```python
from build123d import *

# Parameters (mm, degrees)
SKETCH1_R           = 250
SKETCH1_R_2         = 20
BOSS_EXTRUDE1_DEPTH = 60


with BuildPart() as part:
    # Sketch1 → Boss-Extrude1 (new body)
    with BuildSketch(Plane(origin=(0, 0, 0), x_dir=(0, 0, -1), z_dir=(1, 0, 0))):
        Circle(SKETCH1_R)
        Circle(SKETCH1_R_2, mode=Mode.SUBTRACT)
        with BuildLine():
            Line((177.360116559, 68.142417438), (43.501893686, 24.649244324))
            ThreePointArc((43.501893686, 24.649244324), (29.389262615, 40.450849719), (10, 48.989794856))
            Line((10, 48.989794856), (10, 189.73665961))
            ThreePointArc((10, 189.73665961), (111.679197936, 153.713228931), (177.360116559, 68.142417438))
        make_face(mode=Mode.SUBTRACT)
        with BuildLine():
            Line((-10, 189.73665961), (-10, 48.989794856))
            ThreePointArc((-10, 48.989794856), (-29.389262615, 40.450849719), (-43.501893686, 24.649244324))
            Line((-43.501893686, 24.649244324), (-177.360116559, 68.142417438))
            ThreePointArc((-177.360116559, 68.142417438), (-111.679197936, 153.713228931), (-10, 189.73665961))
        make_face(mode=Mode.SUBTRACT)
        with BuildLine():
            Line((183.540456446, 49.121287113), (49.682233573, 5.628113998))
            ThreePointArc((49.682233573, 5.628113998), (47.552825815, -15.450849719), (36.885648873, -33.755724066))
            Line((36.885648873, -33.755724066), (119.614580282, -147.622329558))
            ThreePointArc((119.614580282, -147.622329558), (180.700738096, -58.713228931), (183.540456446, 49.121287113))
        make_face(mode=Mode.SUBTRACT)
        with BuildLine():
            Line((103.434240394, -159.378034603), (20.705308985, -45.511429112))
            ThreePointArc((20.705308985, -45.511429112), (0, -50), (-20.705308985, -45.511429112))
            Line((-20.705308985, -45.511429112), (-103.434240394, -159.378034603))
            ThreePointArc((-103.434240394, -159.378034603), (0, -190), (103.434240394, -159.378034603))
        make_face(mode=Mode.SUBTRACT)
        with BuildLine():
            Line((-119.614580282, -147.622329558), (-36.885648873, -33.755724066))
            ThreePointArc((-36.885648873, -33.755724066), (-47.552825815, -15.450849719), (-49.682233573, 5.628113998))
            Line((-49.682233573, 5.628113998), (-183.540456446, 49.121287113))
            ThreePointArc((-183.540456446, 49.121287113), (-180.700738096, -58.713228931), (-119.614580282, -147.622329558))
        make_face(mode=Mode.SUBTRACT)
    extrude(amount=BOSS_EXTRUDE1_DEPTH)


solid = part.part
```
Could you check a few things on this model? Use its own coordinates, in mm. A direction names the side the tool comes from. Coordinates: 2 decimals unless noted, no trailing zeros. Order: outer loops, then holes, each group sorted by start corner. A loop starts at its lowest first (then second) coordinate and runs counter-clockwise, first axis right, second up. Notation, with made-up numbers: M -1,-8.75 L 31,-8.75 A14 ccw 31,17.25 Z; hole C 41,14.5 d11. An arc over 180 degrees is marked long. Use one line per item in the form item = value. Start each with the question number.
1. We'd pull the mould along Y, two halves only. Please class faces 3 (the flat face through (0, 59, 3)), 4 (the flat face through (30, 118, -10)): +Y half, -Y half, draft (parallel to the pull), parting line (faces both ways), or undercut.
2. Suppose I cut it at B-B on x = 31.5. Write out the boundary of the cut face in (y, z), then the cut area to 3 significant figures.
3. For pin 1 (6 mm diameter, centred on x = 18, z = 138.5, fed in from -Y); pin 2 (4 mm diameter, centred on x = 9.5, z = -97.5, fed in from -Y); pin 3 (4 mm diameter, centred on x = 19.5, z = -151.5, fed in from +Y), each with a flat end and sliding along its axis, tell me the tip position at first contact or that it passes through.
4. Please list where these lines run through material, in increasing order: line 1 (Y direction, x = 23, z = 0); line 2 (Z direction, x = 34, y = -2); line 3 (Y direction, x = 16.5, z = 147).
5. Suppose I cut it at A-A on z = 0. Write out the boundary of the cut face in (x, y), then the cut area to 3 significant figures.
6. On a 3-axis mill with a long thin cutter (end or side, diameter ignored), from which of +Z, -Z, +X, -X, +Y, -Y can I reach the whole of each face in a straight line? I mean faces 1 (the cylindrical face through (29.58, 40.626, 29.147)), 2 (the flat face through (60, 59, 3)). Say none if no direction works.
7. Suppose I cut it at D-D on z = 97.5. Write out the boundary of the cut face in (x, y), then the cut area to 3 significant figures.
8. Suppose I cut it at C-C on y = 161. Write out the boundary of the cut face in (x, z).
Geometry says:
q1.face_3 = draft
q1.face_4 = undercut
q2.outline = C 0,0 d500; hole M -159.38,-103.43 L -45.51,-20.71 A50 cw -45.51,20.71 L -159.38,103.43 A190 ccw Z; hole M -147.62,-119.61 A190 ccw 49.12,-183.54 L 5.63,-49.68 A50 cw -33.76,-36.89 Z; hole M -147.62,119.61 L -33.76,36.89 A50 cw 5.63,49.68 L 49.12,183.54 A190 ccw Z; hole C 0,0 d40; hole M 24.65,-43.5 L 68.14,-177.36 A190 ccw 189.74,-10 L 48.99,-10 A50 cw Z; hole M 24.65,43.5 A50 cw 48.99,10 L 189.74,10 A190 ccw 68.14,177.36 Z
q2.area = 104,000 mm^2
q3.pin_1 = -210.09
q3.pin_2 = -231.04
q3.pin_3 = 200.37
q4.line_1 = -250 to -190, -50 to -20, 20 to 250
q4.line_2 = -249.99 to -189.99, -49.96 to -19.9, 19.9 to 49.96, 189.99 to 249.99
q4.line_3 = -202.22 to -120.38, 37.25 to 58.28, 120.38 to 202.22
q5.outline = M 0,-250 L 60,-250 L 60,-190 L 0,-190 Z; M 0,-50 L 60,-50 L 60,-20 L 0,-20 Z; M 0,20 L 60,20 L 60,250 L 0,250 Z
q5.area = 19,200 mm^2
q6.face_1 = +X, -X
q6.face_2 = +Z, -Z, +X, +Y, -Y
q7.outline = M 0,-230.2 L 60,-230.2 L 60,-163.08 L 0,-163.08 Z; M 0,-151.21 L 60,-151.21 L 60,-117.18 L 0,-117.18 Z; M 0,21.17 L 60,21.17 L 60,42.19 L 0,42.19 Z; M 0,163.08 L 60,163.08 L 60,230.2 L 0,230.2 Z
q7.area = 11,400 mm^2
q8.outline = M 0,-191.26 L 60,-191.26 L 60,-100.89 L 0,-100.89 Z; M 0,-10 L 60,-10 L 60,10 L 0,10 Z; M 0,100.89 L 60,100.89 L 60,191.26 L 0,191.26 Z
